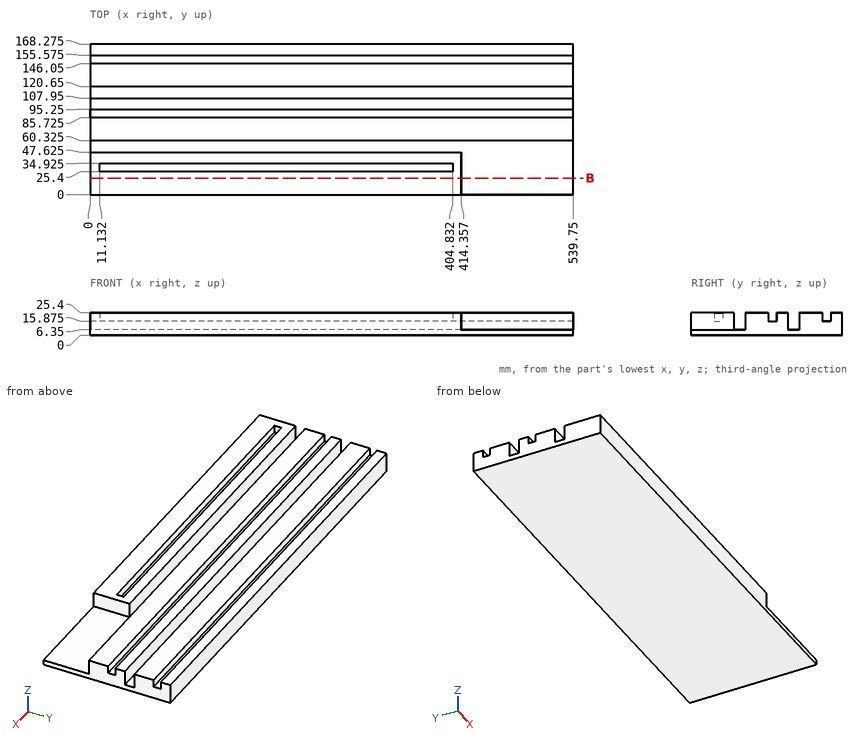
Study the drawing (mm; zero at the part's minimum x, y, z) and answer. Give positions to 0.01 mm unless a question says otherwise; leave off trailing zeros. Order: outer loops, then holes, each group sorted by start corner. A loop starts at its lowest first (then second) coordinate and runs counter-clockwise, first axis right, second up. Notation, with made-up numbers: M -30,47.5 L -24,47.5 A12 ccw -24,65.5 Z; hole C 82,37 d2. An arc over 180 degrees is marked long. Put each result on its own line as item: value. Start each with the question number.
Item 1: Find the intervals of material crossed by line 1 along Z through (x, y) = (185, 59); line 2 along X through (y, z) = (37, 7); line 3 along Z through (x, y) = (348, 90) (1 decimal), in increasing order.
Item 2: Flat-ended cylindrical pins translate along their axes: P1, Ø1, axis at y = 94.5, z = 20.5, coming from the +X side; P2, Ø15, axis at y = 22.5, z = 17, coming from the +X side. Find the tip coordinate at first contact, or state that the pin passes through.
Item 3: The part is cut by section B-B, the plane y = 18.5. Determine the outline of the cut face in (x, z).
Answer key:
1. line 1: z = 0 to 6.35
1. line 2: x = 0 to 414.36
1. line 3: z = 0 to 15.9
2. P1: passes through
2. P2: stops at x = 414.36
3. outline: M 0,0 L 539.75,0 L 539.75,6.35 L 414.36,6.35 L 414.36,25.4 L 0,25.4 Z
